Could you check a few things on this model? Use its own coordinates, in mm. Face numbers are marked on the shaded views. A direction names the side the tool comes from. Coordinates: 2 decimals unless noted, no trailing zeros. Loops run counter-clockwise (first coordinate to the right, second up) from the corner with the lowest first, then second, coordinate; pieces in that order, holes last. Notation, with made-up numbers: (69, 23) - (127, 23) arc R33 ccw to (127, 60) - close; hole circle Ø3 at (1.25, 28.5). An arc over 180 degrees is marked (long way). Put each result on its own line as item: value. Start each with the question number.
```python
from build123d import *

# Parameters (mm, degrees)
SKETCH001_W     = 89
SKETCH001_H     = 14.025192
PAD_DEPTH       = 8
SKETCH002_R     = 3.7
POCKET_DEPTH    = 6
SKETCH003_R     = 1.5
POCKET001_DEPTH = 8.001
SKETCH004_W     = 65
SKETCH004_H     = 4
PAD001_DEPTH    = 25
SKETCH007_W     = 65
SKETCH007_H     = 10.025192
POCKET004_DEPTH = 8
SKETCH008_R     = 1.6
POCKET005_DEPTH = 4
POCKET006_DEPTH = 2.2


with BuildPart() as part:
    # Sketch001 → Pad (new body)
    with BuildSketch(Plane.XY):
        with Locations((126.600648, 156.296259)):
            Rectangle(SKETCH001_W, SKETCH001_H)
    extrude(amount=PAD_DEPTH)

    # Sketch002 (on Face5 of Pad) → Pocket (cut)
    with BuildSketch(Plane(origin=(0, 0, 0), x_dir=(1, 0, 0), z_dir=(0, 0, -1))):
        with Locations((88.100648, -156.408663)):
            Circle(SKETCH002_R)
        with Locations((165.100648, -156.408663)):
            Circle(SKETCH002_R)
    extrude(amount=-POCKET_DEPTH, mode=Mode.SUBTRACT)

    # Sketch003 (on Face6 of Pad) → Pocket001 (cut, through all)
    with BuildSketch(Plane.XY.offset(8)):
        with Locations((88.100648, 156.408663)):
            Circle(SKETCH003_R)
        with Locations((165.100648, 156.408663)):
            Circle(SKETCH003_R)
    extrude(amount=-POCKET001_DEPTH, mode=Mode.SUBTRACT)

    # Sketch004 (on Face5 of Pocket001) → Pad001 (join)
    with BuildSketch(Plane.XY.offset(8)):
        with Locations((126.600648, 161.308855)):
            Rectangle(SKETCH004_W, SKETCH004_H)
    extrude(amount=PAD001_DEPTH)

    # Sketch007 (on Face5 of Pad001) → Pocket004 (cut)
    with BuildSketch(Plane.XY.offset(8)):
        with Locations((126.600648, 154.296259)):
            Rectangle(SKETCH007_W, SKETCH007_H)
    extrude(amount=-POCKET004_DEPTH, mode=Mode.SUBTRACT)

    # Sketch008 (on Face20 of Pocket004) → Pocket005 (cut)
    with BuildSketch(Plane.XZ.offset(-159.308855)):
        with Locations((126.600648, 9)):
            Circle(SKETCH008_R)
        with Locations((126.600648, 23.99)):
            Circle(SKETCH008_R)
    extrude(amount=-POCKET005_DEPTH, mode=Mode.SUBTRACT)

    # Sketch009 (on Face6 of Pocket005) → Pocket006 (cut)
    with BuildSketch(Plane(origin=(0, 163.308855, 0), x_dir=(-1, 0, 0), z_dir=(0, 1, 0))):
        Polygon((-123.800648, 25.606581), (-126.600648, 27.223162), (-129.400648, 25.606581), (-129.400648, 22.373419), (-126.600648, 20.756838), (-123.800648, 22.373419), align=None)
        Polygon((-123.800648, 10.616581), (-126.600648, 12.233162), (-129.400648, 10.616581), (-129.400648, 7.383419), (-126.600648, 5.766838), (-123.800648, 7.383419), align=None)
    extrude(amount=-POCKET006_DEPTH, mode=Mode.SUBTRACT)


solid = part.part
```
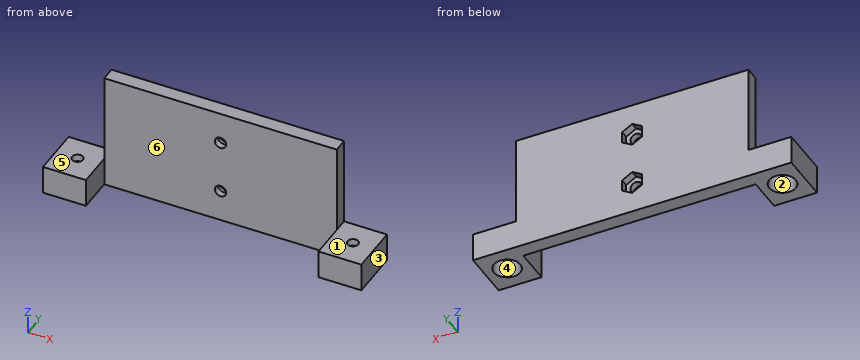
(1) I want a section at B-B on z = 9. List the corners of the cut face in (x, y) for me.
(2) I need wall thicknesses on L1, parallel to X at y = 152.25, z = 3; L2, parallel to X at y = 158.5, z = 3; L3, parallel to X at y = 160.75, z = 24. Which ranges of each line are inside material? Lowest first, please. Write a range as [from, to].
(3) If we mould it in two halves opening along X, with no side actions, what happens to the marked faces 1, 2 and 3? For each: pulls with the +X half, pulls with the -X half, needs draft (parallel to the pull), parting line crosses it, or undercut.
(4) I want a section at C-C on x = 141.5. List the corners of the cut face in (y, z) for me, and give its area (3 significant figures).
(5) I want a section at A-A on y = 151.25. List the corners of the cut face in (x, z) for me, and give its area (3 significant figures).
(6) Which directions (+Z, -Z, +X, -X, +Y, -Y) give clear straight access to the entire face, cutting with the end or side of a thin tool? Please do the marked faces 4, 5 and 6.
(7) For pin 1 Ø3 at (y, z) = (161.5, 11.5) entering from +X; pin 2 Ø4 at (x, y) = (165.1, 156.41) entering from +Z; pin 3 Ø1.7 at (x, z) = (125.5, 10.5) entering from +Y, each with a flat end and sliding along its axis, tell me the tip position at first contact or that it passes through.
Answer sheet:
1. outline: (94.1, 159.31) - (125, 159.31) - (125, 161.11) - (123.8, 161.11) - (123.8, 163.31) - (94.1, 163.31) - close; (128.2, 159.31) - (159.1, 159.31) - (159.1, 163.31) - (129.4, 163.31) - (129.4, 161.11) - (128.2, 161.11) - close
2. L1: x = [82.1, 94.1], [159.1, 171.1]
2. L2: x = [82.1, 85.05], [91.15, 94.1], [159.1, 162.05], [168.15, 171.1]
2. L3: x = [94.1, 125], [128.2, 159.1]
3. face 1: needs draft
3. face 2: undercut
3. face 3: pulls with the +X half
4. outline: (159.31, 0) - (163.31, 0) - (163.31, 33) - (159.31, 33) - close
4. area: 132 mm^2
5. outline: (82.1, 0) - (94.1, 0) - (94.1, 8) - (82.1, 8) - close; (159.1, 0) - (171.1, 0) - (171.1, 8) - (159.1, 8) - close
5. area: 192 mm^2
6. face 4: -Z
6. face 5: +Z, -X, +Y, -Y
6. face 6: +Z, -Z, -Y
7. pin 1: stops at x = 159.1
7. pin 2: stops at z = 8
7. pin 3: stops at y = 161.11
